Work out the finished part from the listing and answer in its coordinate system (mm). Face numbers are marked on the shaded views. A direction names the side the tool comes from. Coordinates: 2 decimals unless noted, no trailing zeros. Order: outer loops, then holes, each group sorted by start corner. A loop starts at its lowest first (then second) coordinate and runs counter-clockwise, first axis right, second up. Notation, with made-up numbers: (53.25, -10.5) -> (104.25, -10.5) arc R24 cw to (104.25, 0.5) -> close; hole circle Ø7 at (-36.5, 4.25). An arc over 180 degrees is marked (long way). Use one line per item in the form item = value.
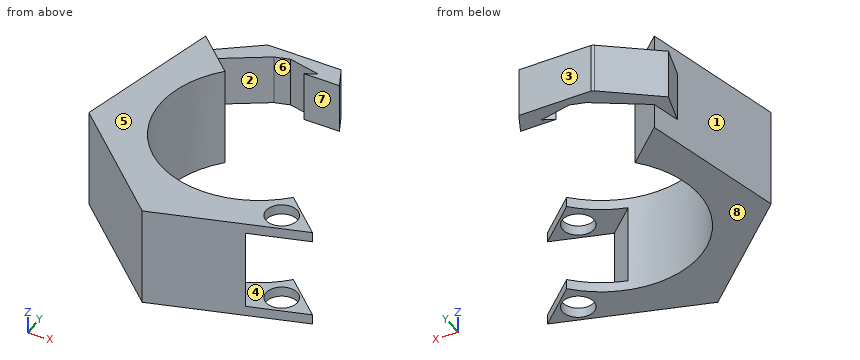
from build123d import *

# Parameters (mm, degrees)
BOSS_EXTRUDE1_DEPTH     = 12.7
CUT_EXTRUDE1_DEPTH      = 10.16
CUT_EXTRUDE2_DEPTH      = 59.972520527
CUT_EXTRUDE2_DEPTH_BACK = 59.972520527
SKETCH3_R               = 4
BOSS_EXTRUDE2_DEPTH     = 6.35


with BuildPart() as part:
    # Sketch1 → Boss-Extrude1 (new, symmetric)
    with BuildSketch(Plane.XY):
        with BuildLine():
            Line((-18.475736443, 16.841827778), (-28.822148851, 26.273251333))
            Line((-28.822148851, 26.273251333), (-37.16437752, -11.82408743))
            Line((-37.16437752, -11.82408743), (-8.342228669, -38.097338763))
            Line((-8.342228669, -38.097338763), (28.822148851, -26.273251333))
            Line((28.822148851, -26.273251333), (18.475736443, -16.841827778))
            ThreePointArc((18.475736443, -16.841827778), (-16.841827778, -18.475736443), (-18.475736443, 16.841827778))
        make_face()
    extrude(amount=BOSS_EXTRUDE1_DEPTH, both=True)

    # Sketch2 → Cut-Extrude1 (cut, symmetric)
    with BuildSketch(Plane.XY):
        Polygon((3.04575912, -20.713698515), (17.349372708, -33.752366684), (38.911165868, -25.491143251), (19.249454098, -2.938003279), align=None)
    extrude(amount=CUT_EXTRUDE1_DEPTH, both=True, mode=Mode.SUBTRACT)

    # Sketch3 → Cut-Extrude2 (cut, two sides: drawn at the far end of the back side and taken through both)
    with BuildSketch(Plane.XY.offset(12.7).offset(-CUT_EXTRUDE2_DEPTH_BACK)):
        with Locations((19.603889038, -24.050389858)):
            Circle(SKETCH3_R)
    extrude(amount=CUT_EXTRUDE2_DEPTH + CUT_EXTRUDE2_DEPTH_BACK, mode=Mode.SUBTRACT)

    # Sketch5 → Boss-Extrude2 (add, symmetric)
    with BuildSketch(Plane.XY):
        Polygon((-30.477907749, 18.711721897), (-32.993263185, 27.186606195), (-19.756729053, 37.411947448), (-19.086323313, 37.739354902), (-0.437878578, 37.739354902), (2.195133213, 32.347949806), (-6.996558268, 32.347949806), (-4.046072735, 33.788884601), (-12.229481166, 35.580817231), (-15.939758745, 34.479602565), (-28.822148851, 26.273251333), align=None)
    extrude(amount=BOSS_EXTRUDE2_DEPTH, both=True)


solid = part.part
(1) Which of the six approach directions +Z, -Z, +X, -X, +Y, -Y give full straight-line access (tool end or side, diameter ignored) to the marked faces 4, 5, 6, 7 and 8?
Data:
face_4 = +X, +Y
face_5 = +Z, +X, -X, +Y, -Y
face_6 = +Z, -Z
face_7 = +Z, -Z, +X
face_8 = -Z, +X, -X, +Y, -Y
(2) Each of these flat-tipped pins is pushed along its axis until it touches: P1, Ø5, axis at x = 17.5, z = -8, coming from the -Y side; P2, Ø21, axis at x = -10.5, y = 33, coming from the +Z side; P3, Ø1, axis at y = 17, z = -1, coming from the -X side. Where does it stop, or does it pass through?
Data:
P1 = -30.28
P2 = 6.35
P3 = -30.96
(3) Section D-D on y = 0 is taken. Write down the section's boundary in (x, z).
Data:
outline = (-34.58, -12.7) -> (-25, -12.7) -> (-25, 12.7) -> (-34.58, 12.7) -> close
(4) Straight lines are drawn through the part: line 1 along Y through (x, z) = (-22.5, -4.25); line 2 along Y through (x, z) = (-3, -4); line 3 along X through (y, z) = (32.5, -2). For each, find the intervals that lie inside material, in ascending order.
Data:
line_1 = -25.19 to -10.9, 10.9 to 20.51, 30.3 to 35.29
line_2 = -36.4 to -24.82, 32.35 to 37.74
line_3 = -26.12 to -19.05, -6.69 to 2.12
(5) The mould has two halves that part along X. Classify the marked faces 1, 2 and 3: released by +X, released by -X, zero draft, split by the parting line, or undercut.
Data:
face_1 = released by -X
face_2 = undercut
face_3 = zero draft
(6) Section B-B on y = 25 is taken. Write down the section's boundary in (x, z).
Data:
outline = (-32.34, -6.35) -> (-29.1, -6.35) -> (-29.1, -12.7) -> (-27.43, -12.7) -> (-27.43, 12.7) -> (-29.1, 12.7) -> (-29.1, 6.35) -> (-32.34, 6.35) -> close
(7) Section C-C on y = 8.5 is taken. Write down the section's boundary in (x, z).
Data:
outline = (-32.71, -12.7) -> (-23.51, -12.7) -> (-23.51, 12.7) -> (-32.71, 12.7) -> close
(8) Section A-A on x = 21 is taken. Write down the section's boundary in (y, z), plus the area to 3 significant figures.
Data:
outline = (-28.76, -12.7) -> (-27.8, -12.7) -> (-27.8, -10.16) -> (-28.76, -10.16) -> close; (-28.76, 10.16) -> (-27.8, 10.16) -> (-27.8, 12.7) -> (-28.76, 12.7) -> close; (-20.3, -12.7) -> (-19.14, -12.7) -> (-19.14, -10.16) -> (-20.3, -10.16) -> close; (-20.3, 10.16) -> (-19.14, 10.16) -> (-19.14, 12.7) -> (-20.3, 12.7) -> close
area = 10.8 mm²
